Read the model definition and answer for the solid it produces. Units are mm, in the model's axes. Face numbers are marked on the shaded views. Coordinates: 2 decimals unless noted, no trailing zeros. Write each loop counter-clockwise with the first axis right and the second up, starting at its lowest first coordinate (ties: lowest second). Pieces come first, ordered by that corner, then holes. Notation, with made-up numbers: (-13.75, 12) -> (-0.75, 12) arc R16 cw to (-0.75, 32) -> close; hole circle Ø3 at (-16.75, 41.5). An arc over 180 degrees is marked (long way). Return JSON: item names as keys, results as strings.
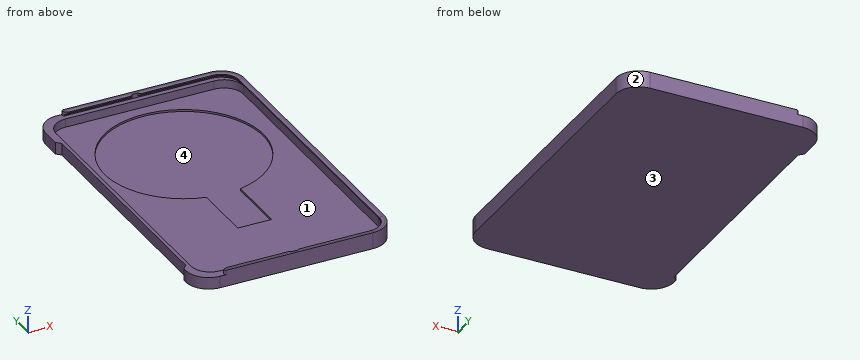
from build123d import *

# Parameters (mm, degrees)
PAD_DEPTH       = 1.6
PAD_DEPTH_BACK  = 4.2
POCKET001_DEPTH = 3
POCKET002_DEPTH = 10
POCKET003_DEPTH = 3.7
POCKET_DEPTH    = 5


with BuildPart() as part:
    # Sketch → Pad (new body, two sides)
    with BuildSketch(Plane.XY) as pad_sk:
        with BuildLine():
            ThreePointArc((-6, 2), (-3.656854, -3.656854), (2, -6))
            Line((56, -6), (2, -6))
            ThreePointArc((56, -6), (61.656854, -3.656854), (64, 2))
            Line((64, 99), (64, 2))
            ThreePointArc((64, 99), (61.656854, 104.656854), (56, 107))
            Line((2, 107), (56, 107))
            ThreePointArc((2, 107), (-3.656854, 104.656854), (-6, 99))
            Line((-6, 92.3), (-6, 99))
            Line((-6, 92.3), (-4.5, 90.8))
            Line((-4.5, 90.8), (-4.5, 5))
            Line((-6, 3.5), (-4.5, 5))
            Line((-6, 2), (-6, 3.5))
        make_face()
    extrude(amount=PAD_DEPTH)
    extrude(pad_sk.sketch, amount=-PAD_DEPTH_BACK)

    # Sketch002 → Pocket001 (cut)
    with BuildSketch(Plane.XY):
        with BuildLine():
            ThreePointArc((3.5, 104), (-1.308326, 102.008326), (-3.3, 97.2))
            Line((-3.3, 3.8), (-3.3, 97.2))
            ThreePointArc((-3.3, 3.8), (-1.308326, -1.008326), (3.5, -3))
            Line((56, -3), (3.5, -3))
            ThreePointArc((56, -3), (60.808326, -1.008326), (62.8, 3.8))
            Line((62.8, 97.2), (62.8, 3.8))
            ThreePointArc((62.8, 97.2), (60.808326, 102.008326), (56, 104))
            Line((3.5, 104), (56, 104))
        make_face()
    extrude(amount=-POCKET001_DEPTH, mode=Mode.SUBTRACT)

    # Sketch003 → Pocket002 (cut)
    with BuildSketch(Plane.XY):
        Polygon((24.9, -1.8), (24.9, 102.8), (27.9, 105.8), (30.1, 105.8), (33.1, 102.8), (33.1, -1.8), (30.1, -4.8), (27.9, -4.8), align=None)
        with BuildLine():
            Line((3.93923, 105.880385), (5.117691, 105.2))
            Line((5.117691, 105.2), (-11.76077, 105.2))
            Line((-11.76077, 107), (-11.76077, 105.2))
            Line((4.23923, 107), (-11.76077, 107))
            ThreePointArc((4.23923, 107), (3.659675, 106.555291), (3.93923, 105.880385))
        make_face()
        with BuildLine():
            Line((3.93923, -4.880385), (5.117691, -4.2))
            Line((5.117691, -4.2), (-11.76077, -4.2))
            Line((-11.76077, -4.2), (-11.76077, -6))
            Line((-11.76077, -6), (4.23923, -6))
            ThreePointArc((3.93923, -4.880385), (3.659675, -5.555291), (4.23923, -6))
        make_face()
    extrude(amount=POCKET002_DEPTH, mode=Mode.SUBTRACT)

    # Sketch004 → Pocket003 (cut)
    with BuildSketch(Plane.XY):
        with BuildLine():
            ThreePointArc((35, 44.650411), (29, 100), (23, 44.650411))
            Line((23, 23), (23, 44.650411))
            Line((35, 23), (23, 23))
            Line((35, 44.650411), (35, 23))
        make_face()
    extrude(amount=-POCKET003_DEPTH, mode=Mode.SUBTRACT)

    # SubtractivePipe: sweep along a path in Sketch005
    with BuildLine(Plane.XY) as subtractivepipe_path:
        Line((-6, -6), (56, -6))
        ThreePointArc((56, -6), (61.656854, -3.656854), (64, 2))
        Line((64, 2), (64, 99))
        ThreePointArc((64, 99), (61.656854, 104.656854), (56, 107))
        Line((56, 107), (-6, 107))
    # Sketch001 → SubtractivePipe (sweep, cut)
    with BuildSketch(Plane.YZ):
        Polygon((-4.8, 0), (-4.8, 0.4), (-4.2, 1), (-4.2, 1.4), (-5.334256, 1.6), (-3.334256, 1.6), (-3.334256, 0), align=None)
    sweep(path=subtractivepipe_path.line, mode=Mode.SUBTRACT)

    # Sketch006 → Pocket (cut)
    with BuildSketch(Plane.XY):
        with BuildLine():
            Line((-6, -4), (56, -4))
            ThreePointArc((56, -4), (60.242641, -2.242641), (62, 2))
            Line((62, 2), (62, 99))
            ThreePointArc((62, 99), (60.242641, 103.242641), (56, 105))
            Line((56, 105), (-6, 105))
            Line((-6, 105), (-6, -4))
        make_face()
    extrude(amount=POCKET_DEPTH, mode=Mode.SUBTRACT)


solid = part.part
1. The part is cut by section D-D (x = 29). Determine the outline of the cut face in (y, z).
Taken from the geometry:
{"outline": "(-6, -4.2) -> (107, -4.2) -> (107, 1.6) -> (106.33, 1.6) -> (105.8, 1.51) -> (105.8, 0) -> (104, 0) -> (104, -3) -> (100, -3) -> (100, -3.7) -> (23, -3.7) -> (23, -3) -> (-3, -3) -> (-3, 0) -> (-4.8, 0) -> (-4.8, 1.51) -> (-5.33, 1.6) -> (-6, 1.6) -> close"}
2. The part is cut by section B-B (x = 49). Determine the outline of the cut face in (y, z), then the cut area to 3 significant figures.
Taken from the geometry:
{"outline": "(-6, -4.2) -> (107, -4.2) -> (107, 1.6) -> (106.33, 1.6) -> (105.2, 1.4) -> (105.2, 1) -> (105.8, 0.4) -> (105.8, 0) -> (104, 0) -> (104, -3) -> (91.6, -3) -> (91.6, -3.7) -> (52.4, -3.7) -> (52.4, -3) -> (-3, -3) -> (-3, 0) -> (-4.8, 0) -> (-4.8, 0.4) -> (-4.2, 1) -> (-4.2, 1.4) -> (-5.33, 1.6) -> (-6, 1.6) -> close", "area": "131 mm2"}
3. For a pull along X with two mould halves and no side action, classify the marked faces 1, 2, 3 and 4 as +X half, -X half, draft (parallel to the pull), parting line (faces both ways), or undercut.
Taken from the geometry:
{"face 1": "undercut", "face 2": "+X half", "face 3": "draft", "face 4": "undercut"}
4. The part is cut by section C-C (y = 18). Determine the outline of the cut face in (x, z), then the cut area to 3 significant figures.
Taken from the geometry:
{"outline": "(-4.5, -4.2) -> (64, -4.2) -> (64, 1.6) -> (63.33, 1.6) -> (62.2, 1.4) -> (62.2, 1) -> (62.8, 0.4) -> (62.8, -3) -> (-3.3, -3) -> (-3.3, 0) -> (-4.5, 0) -> close", "area": "91.7 mm2"}
5. The part is cut by section A-A (y = 72). Determine the outline of the cut face in (x, z), then the cut area to 3 significant figures.
Taken from the geometry:
{"outline": "(-4.5, -4.2) -> (64, -4.2) -> (64, 1.6) -> (63.33, 1.6) -> (62.2, 1.4) -> (62.2, 1) -> (62.8, 0.4) -> (62.8, -3) -> (57, -3) -> (57, -3.7) -> (1, -3.7) -> (1, -3) -> (-3.3, -3) -> (-3.3, 0) -> (-4.5, 0) -> close", "area": "52.5 mm2"}
6. Flat-ended cylindrical pins translate along their axes: pin 1 Ø1.7 at (y, z) = (57, -1) entering from -X; pin 2 Ø6 at (x, y) = (13, 88.5) entering from +Z. Find the tip coordinate at first contact, or state that the pin passes through.
Taken from the geometry:
{"pin 1": "stops at x = -4.5", "pin 2": "stops at z = -3.7"}
7. Consider L1, parallel to X at y = 72, z = -3.4; L2, parallel to Y at x = 29, z = -3.5; L3, parallel to X at y = 77.5, z = -0.45. Determine where each line is inside the solid, lowest interval first.
Taken from the geometry:
{"L1": "x = -4.5 to 1, 57 to 64", "L2": "y = -6 to 23, 100 to 107", "L3": "x = -4.5 to -3.3, 62.8 to 64"}
